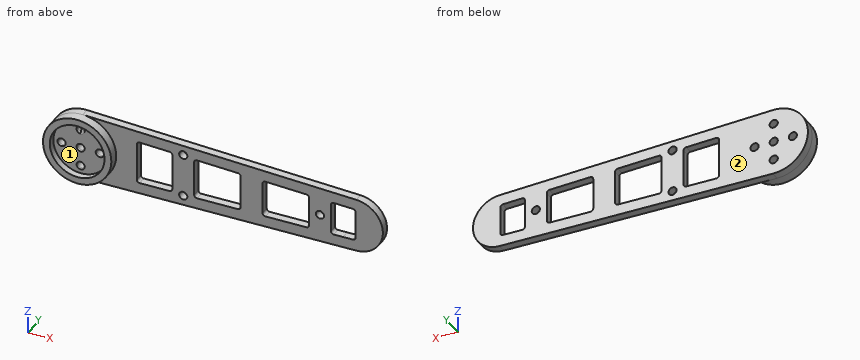
```python
from build123d import *
from build123d.topology import SkipClean

# Parameters (mm, degrees)
SKETCH_1_R          = 1.5
EXTRUDE_1_DEPTH     = 3
EXTRUDE_START       = 3.5
SKETCH_2_R          = 12.5
SKETCH_2_R_2        = 10
EXTRUDE_2_DEPTH     = 3.5
CUT_EXTRUDE_1_DEPTH = 10
FILLET_1_R          = 1
EXTRUDE_START_2     = 1
SKETCH_5_R          = 10
SKETCH_5_R_2        = 1.5
EXTRUDE_3_DEPTH     = 1


with BuildPart() as part:
    # 草图1 → 凸台-拉伸1 (new body)
    with BuildSketch(Plane(origin=(0, 0, 0), x_dir=(1, 0, 0), z_dir=(0, 1, 0))):
        with BuildLine():
            Line((100.25, 9.996874512), (0.3125, 12.496093139))
            ThreePointArc((0.3125, 12.496093139), (-12.5, 0), (0.3125, -12.496093139))
            Line((0.3125, -12.496093139), (100.25, -9.996874512))
            ThreePointArc((100.25, -9.996874512), (110, 0), (100.25, 9.996874512))
        make_face()
        with Locations(Location((7, 0, 0), (0, 0, 270))):
            Circle(SKETCH_1_R, mode=Mode.SUBTRACT)
        with Locations(Location((0, 0, 0), (0, 0, 270))):
            Circle(SKETCH_1_R, mode=Mode.SUBTRACT)
        with Locations(Location((-7, 0, 0), (0, 0, 270))):
            Circle(SKETCH_1_R, mode=Mode.SUBTRACT)
        with Locations(Location((0, 7, 0), (0, 0, 270))):
            Circle(SKETCH_1_R, mode=Mode.SUBTRACT)
        with Locations(Location((0, -7, 0), (0, 0, 270))):
            Circle(SKETCH_1_R, mode=Mode.SUBTRACT)
    extrude(amount=EXTRUDE_1_DEPTH)

    # 草图2 → 凸台-拉伸2 (add)
    with BuildSketch(Plane.XZ.offset(EXTRUDE_START)):
        with Locations(Location((0, 0, 0), (0, 0, 270))):
            Circle(SKETCH_2_R)
        with Locations(Location((0, 0, 0), (0, 0, 270))):
            Circle(SKETCH_2_R_2, mode=Mode.SUBTRACT)
    extrude(amount=-EXTRUDE_2_DEPTH)

    # 草图3 → 切除-拉伸1 (cut)
    with BuildSketch(Plane(origin=(0, 3, 0), x_dir=(1, 0, 0), z_dir=(0, 1, 0))):
        Polygon((20, 8.002501172), (20, 0), (33, 0), (33, 7.677399562), align=None)
        Polygon((33, 0), (20, 0), (20, -8.002501172), (33, -7.677399562), align=None)
        with BuildLine():
            ThreePointArc((38.5, 8), (36.805156295, 9.487291475), (35.550618759, 7.613614157))
            Line((35.550618759, 7.613614157), (38.42825626, 7.541650728))
            ThreePointArc((38.42825626, 7.541650728), (38.481955531, 7.768034906), (38.5, 8))
        make_face()
        with BuildLine():
            Line((38.42825626, 7.541650728), (35.550618759, 7.613614157))
            ThreePointArc((35.550618759, 7.613614157), (36.9625, 6.500468823), (38.42825626, 7.541650728))
        make_face()
        with BuildLine():
            ThreePointArc((38.42825626, -7.541650728), (36.9625, -6.500468823), (35.550618759, -7.613614157))
            Line((35.550618759, -7.613614157), (38.42825626, -7.541650728))
        make_face()
        with BuildLine():
            Line((38.42825626, -7.541650728), (35.550618759, -7.613614157))
            ThreePointArc((35.550618759, -7.613614157), (36.805156295, -9.487291475), (38.5, -8))
            ThreePointArc((38.5, -8), (38.481955531, -7.768034906), (38.42825626, -7.541650728))
        make_face()
        Polygon((41, 7.477337033), (41, 0), (58, 0), (58, 7.052204158), align=None)
        Polygon((58, 0), (41, 0), (41, -7.477337033), (58, -7.052204158), align=None)
        Polygon((66, 6.852141629), (66, 0), (83, 0), (83, 6.427008754), align=None)
        Polygon((83, 0), (66, 0), (66, -6.852141629), (83, -6.427008754), align=None)
        with BuildLine():
            ThreePointArc((88.5, 0), (87, 1.5), (85.5, 0))
            Line((85.5, 0), (88.5, 0))
        make_face()
        with BuildLine():
            Line((88.5, 0), (85.5, 0))
            ThreePointArc((85.5, 0), (87, -1.5), (88.5, 0))
        make_face()
        Polygon((95.393745853, 6.117068236), (91, 6.226946225), (91, 0), (100, 0), (100, 6.001875879), align=None)
        Polygon((91, 0), (91, -6.226946225), (100, -6.001875879), (100, 0), align=None)
    extrude(amount=-CUT_EXTRUDE_1_DEPTH, mode=Mode.SUBTRACT)

    # 圆角1
    fillet_1_edges = [part.edges().sort_by_distance(p)[0] for p in [
        (91, 1.5, 6.226946225),
        (91, 1.5, -6.226946225),
        (100, 1.5, -6.001875879),
        (100, 1.5, 6.001875879),
        (20, 1.5, 8.002501172),
        (20, 1.5, -8.002501172),
        (33, 1.5, -7.677399562),
        (33, 1.5, 7.677399562),
        (41, 1.5, 7.477337033),
        (41, 1.5, -7.477337033),
        (58, 1.5, -7.052204158),
        (58, 1.5, 7.052204158),
        (66, 1.5, 6.852141629),
        (66, 1.5, -6.852141629),
        (83, 1.5, -6.427008754),
        (83, 1.5, 6.427008754),
    ]]
    fillet(fillet_1_edges, radius=FILLET_1_R)

    # 草图5 → 凸台-拉伸3 (add)
    with SkipClean():  # the faces are left unmerged after this step: merging them gives an invalid solid
        with BuildSketch(Plane.XZ.offset(EXTRUDE_START_2)):
            with Locations(Location((0, 0, 0), (0, 0, 270))):
                Circle(SKETCH_5_R)
            with Locations(Location((0, 0, 0), (0, 0, 270))):
                Circle(SKETCH_5_R_2, mode=Mode.SUBTRACT)
            with Locations(Location((7, 0, 0), (0, 0, 270))):
                Circle(SKETCH_5_R_2, mode=Mode.SUBTRACT)
            with Locations(Location((-7, 0, 0), (0, 0, 270))):
                Circle(SKETCH_5_R_2, mode=Mode.SUBTRACT)
            with Locations(Location((0, -7, 0), (0, 0, 270))):
                Circle(SKETCH_5_R_2, mode=Mode.SUBTRACT)
            with Locations(Location((0, 7, 0), (0, 0, 270))):
                Circle(SKETCH_5_R_2, mode=Mode.SUBTRACT)
        extrude(amount=-EXTRUDE_3_DEPTH)


solid = part.part
```
Input: part model. Units: mm. Frame: model coordinates. Face numbers are marked on the shaded views. Give positions to 0.01 mm unless a question says otherwise; leave off trailing zeros. Order: outer loops, then holes, each group sorted by start corner. A loop starts at its lowest first (then second) coordinate and runs counter-clockwise, first axis right, second up. Notation, with made-up numbers: (-25, 59.5) - (28, 59.5) arc R37 cw to (28, 97.5) - close; hole circle Ø2 at (0, -20.75). An arc over 180 degrees is marked (long way). Use a Markdown table: item, result.
(1) Section query B-B (x = 37). Output: boundary loops of the cut face in (y, z).
Computed values:
| item | result |
|---|---|
| outline | (0, -11.58) - (3, -11.58) - (3, -9.5) - (0, -9.5) - close; (0, -6.5) - (3, -6.5) - (3, 6.5) - (0, 6.5) - close; (0, 9.5) - (3, 9.5) - (3, 11.58) - (0, 11.58) - close |
(2) Line query: line 1 (X direction, y = -0.2, z = 0); line 2 (Z direction, x = 37, y = 1.2). Output: solid intervals per line, ascending. Write a range as from..to.
Computed values:
| item | result |
|---|---|
| line 1 | x = -12.5..-8.5, -5.5..-1.5, 1.5..5.5, 8.5..12.5 |
| line 2 | z = -11.58..-9.5, -6.5..6.5, 9.5..11.58 |
(3) Section query A-A (x = 87). Output: boundary loops of the cut face in (y, z), then the cut area to 3 significant figures.
Computed values:
| item | result |
|---|---|
| outline | (0, -10.33) - (3, -10.33) - (3, -1.5) - (0, -1.5) - close; (0, 1.5) - (3, 1.5) - (3, 10.33) - (0, 10.33) - close |
| area | 53.0 mm2 |
(4) Draft query along Z for the marked faces 1 and 2. Return one class per face: released by +Z, released by -Z, zero draft, split by the parting line, or undercut.
Computed values:
| item | result |
|---|---|
| face 1 | undercut |
| face 2 | zero draft |
(5) Pin query (flat end, axial travel): pin 1 (2.5 mm diameter, centred on y = 1.5, z = 1.5, fed in from -X); pin 2 (3.5 mm diameter, centred on x = 87, z = 0, fed in from -Y); pin 3 (2.5 mm diameter, centred on x = 0, z = -7, fed in from -Y); pin 4 (1.5 mm diameter, centred on x = 59.5, y = 0.5, fed in from +Z). Return the tip coordinate at first contact, or that it passes through.
Computed values:
| item | result |
|---|---|
| pin 1 | stops at x = -12.5 |
| pin 2 | stops at y = 0 |
| pin 3 | passes through |
| pin 4 | stops at z = 11.03 |
(6) Section query C-C (z = 0). State how many separate pieces and enclosed holes the cut face has, then the cut area to 3 significant figures.
Computed values:
| item | result |
|---|---|
| separate pieces | 9 |
| enclosed holes | 0 |
| area | 192 mm2 |
